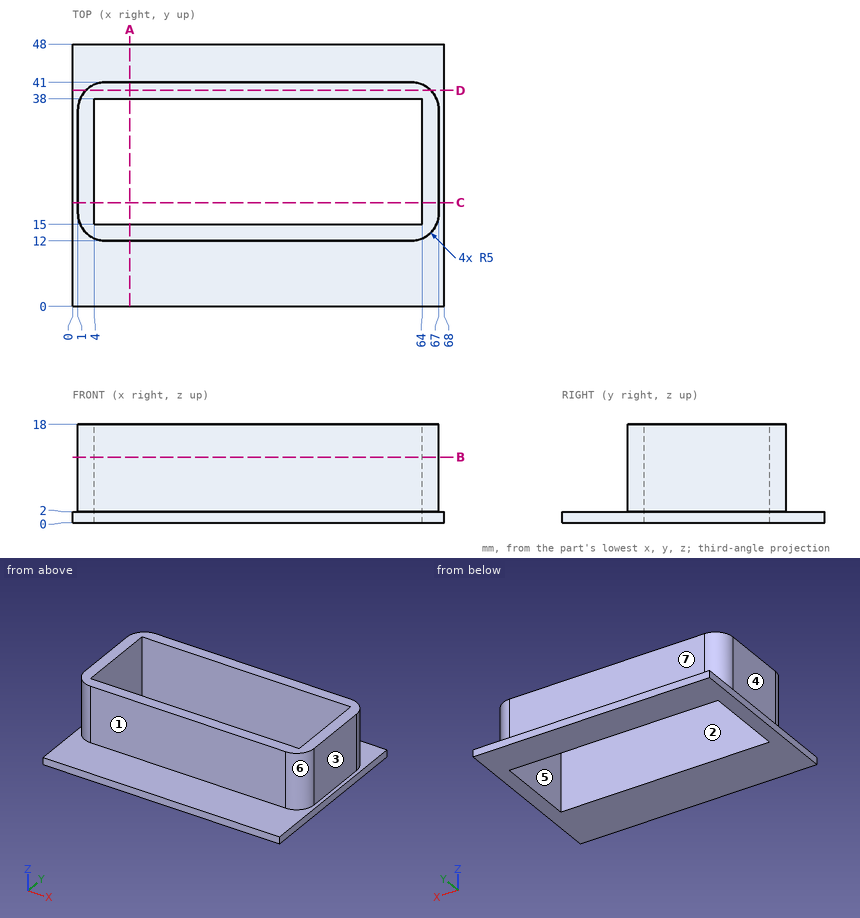
Verification items for this drawing (mm, ordinates from the low corner). A direction names the side the tool comes from. Coordinates: 2 decimals unless noted, no trailing zeros. Loops run counter-clockwise (first coordinate to the right, second up) from the corner with the lowest first, then second, coordinate; pieces in that order, holes last.
Item 1: Access from +Z, -Z, +X, -X, +Y, -Y to the whole of each face (thin tool, end or side, straight path). Record for the marked faces 1, 2, 3 and 4.
Item 2: Sectioned sample at C-C, the plane y = 19. Record the boundary of the cut face in (x, z), then the cut area to 3 significant figures.
Item 3: Sectioned sample at B-B, the plane z = 12. Record the boundary of the cut face in (x, y).
Item 4: Thickness scan on line 1 (Y direction, x = 9, z = 12); line 2 (X direction, y = 26, z = 17.25); line 3 (Y direction, x = 11.5, z = 1). Record the ranges inside material, lowest first.
Item 5: Sectioned sample at A-A, the plane x = 10.5. Record the boundary of the cut face in (y, z).
Item 6: Sectioned sample at D-D, the plane y = 39.5. Record the boundary of the cut face in (x, z), then the cut area to 3 significant figures.
Item 7: Release check for a two-part mould opening along X. For the marked faces 5, 6 and 7 record: released by +X, released by -X, zero draft, split by the parting line, or undercut.
Item 8: Go/stop test with flat-tipped pins: pin 1 Ø3 at (y, z) = (31.5, 9.5) entering from -X; pin 2 Ø1.5 at (x, z) = (50.5, 8.5) entering from -Y; pin 3 Ø1.5 at (y, z) = (17, 5.5) entering from +X. Record where each tip stops, or that it passes through.
Check result:
1. face 1: +Z, +X, -X, -Y
1. face 2: +Z, -Z
1. face 3: +Z, +X, +Y, -Y
1. face 4: +Z, -X, +Y, -Y
2. outline: (0, 0) - (4, 0) - (4, 18) - (1, 18) - (1, 2) - (0, 2) - close; (64, 0) - (68, 0) - (68, 2) - (67, 2) - (67, 18) - (64, 18) - close
2. area: 112 mm2
3. outline: (1, 17) arc R5 ccw to (6, 12) - (62, 12) arc R5 ccw to (67, 17) - (67, 36) arc R5 ccw to (62, 41) - (6, 41) arc R5 ccw to (1, 36) - close; hole (4, 15) - (64, 15) - (64, 38) - (4, 38) - close
4. line 1: y = 12 to 15, 38 to 41
4. line 2: x = 1 to 4, 64 to 67
4. line 3: y = 0 to 15, 38 to 48
5. outline: (0, 0) - (15, 0) - (15, 18) - (12, 18) - (12, 2) - (0, 2) - close; (38, 0) - (48, 0) - (48, 2) - (41, 2) - (41, 18) - (38, 18) - close
6. outline: (0, 0) - (68, 0) - (68, 2) - (65.57, 2) - (65.57, 18) - (2.43, 18) - (2.43, 2) - (0, 2) - close
6. area: 1,150 mm2
7. face 5: undercut
7. face 6: released by +X
7. face 7: zero draft
8. pin 1: stops at x = 1
8. pin 2: stops at y = 12
8. pin 3: stops at x = 67
